from build123d import *

# Parameters (mm, degrees)
F0_R      = 6
F1_DEPTH  = 450
F2_SIZE   = 2
F4_R      = 12.5
F5_DEPTH  = 10
F6_SIZE   = 2
F8_DEPTH  = 5
F10_D     = 12
F10_DEPTH = 30


with BuildPart() as f1:
    # F0 (on Front) → F1 (new body)
    with BuildSketch(Plane.XZ):
        Circle(F0_R)
    extrude(amount=F1_DEPTH)

    # F2
    f2_edges = [f1.edges().sort_by_distance(p)[0] for p in [
        (-6, -450, 0),
        (-6, 0, 0),
    ]]
    chamfer(f2_edges, length=F2_SIZE)

    # F4 (on offset) → F5 (join, symmetric)
    with BuildSketch(Plane.XZ.offset(225)):
        Circle(F4_R)
    extrude(amount=F5_DEPTH, both=True)

    # F6
    f6_edges = [f1.edges().sort_by_distance(p)[0] for p in [
        (-12.5, -235, 0),
        (-12.5, -215, 0),
    ]]
    chamfer(f6_edges, length=F6_SIZE)

    # F7 (on offset) → F8 (join, symmetric)
    with BuildSketch(Plane.XZ.offset(225)):
        with BuildLine():
            ThreePointArc((19.879044, 2.196272), (1e-06, 20), (-19.879044, 2.196273))
            ThreePointArc((-19.879044, 2.196273), (-1.099801, -19.969738), (20, 0))
            ThreePointArc((20, 0), (19.969738, 1.0998), (19.879044, 2.196272))
        make_face()
        with BuildLine():
            Line((-12.432798, 69.594193), (-19.879044, 2.196273))
            ThreePointArc((-19.879044, 2.196273), (1e-06, 20), (19.879044, 2.196272))
            Line((19.879044, 2.196272), (12.432798, 69.594193))
            ThreePointArc((12.432798, 69.594193), (12.483188, 68.947853), (12.5, 68.29977))
            ThreePointArc((12.5, 68.29977), (-0.648083, 55.816582), (-12.432798, 69.594193))
        make_face()
        with BuildLine():
            ThreePointArc((12.432798, 69.594193), (0, 80.79977), (-12.432798, 69.594193))
            ThreePointArc((-12.432798, 69.594193), (-0.648083, 55.816582), (12.5, 68.29977))
            ThreePointArc((12.5, 68.29977), (12.483188, 68.947853), (12.432798, 69.594193))
        make_face()
    extrude(amount=F8_DEPTH, both=True)

    # F10
    with Locations(Plane.XZ.offset(230)):
        with Locations((0, 68.29977)):
            Hole(F10_D / 2, depth=F10_DEPTH)


solid = f1.part
Source: CAD feature listing. Evaluate the final solid. Frame: model axes, mm. A direction names the side the tool comes from. Coordinates: 2 decimals unless noted, no trailing zeros. Loops run counter-clockwise (first coordinate to the right, second up) from the corner with the lowest first, then second, coordinate; pieces in that order, holes last. Notation, with made-up numbers: (76, 53) -> (81, 53) arc R22 ccw to (81, 69) -> close; hole circle Ø6 at (80.5, 54.25). An arc over 180 degrees is marked (long way). Answer in a Markdown table with one row per item. Add a question column.
Q1. Contact query for flat-ended pins moving along their axis: pin 1 Ø5 at (x, y) = (-4.5, -325) entering from -Z; pin 2 Ø10 at (x, z) = (-13, 42.5) entering from -Y; pin 3 Ø12 at (x, z) = (12, 60) entering from +Y; pin 4 Ø7 at (x, z) = (0, 68.3) entering from -Y. Output: stop coordinate, or through.
Q2. Pull-direction query (X, two-part tool) for faces 4 (the face through (0, -450, 0)), 5 (the face through (0.78, -224.93, 74.25)), 6 (the face through (-16.1, -225.1, 36.4)); classes: pulls with the +X half, pulls with the -X half, needs draft (parallel to the pull), parting line crosses it, or undercut.
Q3. Section B-B on y = -141. Return the cut outline in (x, z), and give its area (3 significant figures).
Q4. Section C-C on z = 47.5. Return the cut outline in (x, y), and give its area (3 significant figures).
Q5. Ray query, line 1 along Z through (x, y) = (0, -226.5); line 2 along Y through (x, z) = (-5, 31); line 3 along Z through (x, y) = (2, -298). Return the intervals inside material, ascending.
Q6. Reachability of faces 1 (the face through (5, -235, -5)), 2 (the face through (0.257, -225.07, 80.797)), 3 (the face through (5, -215, -5)) from +Z, -Z, +X, -X, +Y, -Y: full face, straight path, thin tool, end or side. Return the list, or none.
Computed values:
| question | item | result |
|---|---|---|
| 1 | pin 1 | stops at z = -5.66 |
| 1 | pin 2 | stops at y = -230 |
| 1 | pin 3 | stops at y = -220 |
| 1 | pin 4 | passes through |
| 2 | face 4 | needs draft |
| 2 | face 5 | undercut |
| 2 | face 6 | pulls with the -X half |
| 3 | outline | circle Ø12 at (0, 0) |
| 3 | area | 113 mm^2 |
| 4 | outline | (-14.87, -230) -> (14.87, -230) -> (14.87, -220) -> (-14.87, -220) -> close |
| 4 | area | 297 mm^2 |
| 5 | line 1 | z = -20 to 62.3, 74.3 to 80.8 |
| 5 | line 2 | y = -230 to -220 |
| 5 | line 3 | z = -5.66 to 5.66 |
| 6 | face 1 | -Y |
| 6 | face 2 | +Z, +Y, -Y |
| 6 | face 3 | +Y |
